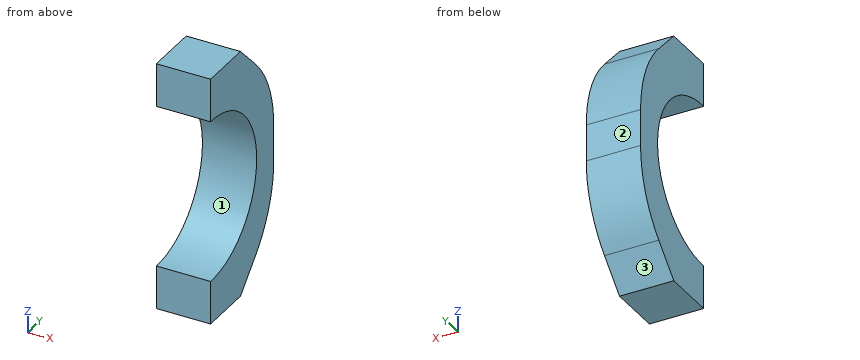
from build123d import *

# Parameters (mm, degrees)
BOSS_EXTRUDE1_DEPTH = 12
CHAMFER1_SIZE       = 16
FILLET1_R           = 30
BOSS_EXTRUDE3_DEPTH = 15


with BuildPart() as part:
    # Sketch1 → Boss-Extrude1 (new body)
    with BuildSketch(Plane(origin=(0, 0, 0), x_dir=(0, 0, -1), z_dir=(1, 0, 0))):
        with BuildLine():
            Line((-33.494680249, 0), (33.494680249, 0))
            Line((33.494680249, 0), (33.494680249, -29.5))
            Line((33.494680249, -29.5), (23.494680249, -29.5))
            ThreePointArc((23.494680249, -29.5), (0, -6.5), (-23.494680249, -29.5))
            Line((-23.494680249, -29.5), (-33.494680249, -29.5))
            Line((-33.494680249, -29.5), (-33.494680249, 0))
        make_face()
    extrude(amount=BOSS_EXTRUDE1_DEPTH)

    # Chamfer1
    chamfer1_edges = [part.edges().sort_by_distance(p)[0] for p in [
        (6, 0, 33.494680249),
        (6, 0, -33.494680249),
    ]]
    chamfer(chamfer1_edges, length=CHAMFER1_SIZE)

    # Fillet1
    fillet1_edges = [part.edges().sort_by_distance(p)[0] for p in [
        (6, 0, 17.494680249),
        (6, 0, -17.494680249),
    ]]
    fillet(fillet1_edges, radius=FILLET1_R)

    # Sketch6 → Boss-Extrude3 (add)
    with BuildSketch(Plane(origin=(12, 0, 0), x_dir=(0, 0, -1), z_dir=(1, 0, 0))):
        with BuildLine():
            Line((34.494680249, -15.585786438), (26.988583595, -8.079689783))
            ThreePointArc((26.988583595, -8.079689783), (16.931459781, -1.359734492), (5.068273378, 1))
            Line((5.068273378, 1), (-5.068273378, 1))
            ThreePointArc((-5.068273378, 1), (-16.931459781, -1.359734492), (-26.988583595, -8.079689783))
            Line((-26.988583595, -8.079689783), (-34.494680249, -15.585786438))
            Line((-34.494680249, -15.585786438), (-34.494680249, -30.5))
            Line((-34.494680249, -30.5), (-22.494443758, -30.5))
            ThreePointArc((-22.494443758, -30.5), (0, -7.5), (22.494443758, -30.5))
            Line((22.494443758, -30.5), (34.494680249, -30.5))
            Line((34.494680249, -30.5), (34.494680249, -15.585786438))
        make_face()
    extrude(amount=-BOSS_EXTRUDE3_DEPTH)


solid = part.part
Check sheet for the modelled part. Datum: model origin and axes. Units: mm. Face numbers are marked on the shaded views. Give positions to 0.01 mm unless a question says otherwise; leave off trailing zeros. Loops run counter-clockwise (first coordinate to the right, second up) from the corner with the lowest first, then second, coordinate; pieces in that order, holes last. Notation, with made-up numbers: M 87,48.5 L 139,48.5 A13 ccw 139,58.5 Z; hole C 28.25,17.25 d10. An arc over 180 degrees is marked long. Answer as a JSON object with one key per item and string values. Group by question number.
Q1. Material ranges on line 1 along Z through (x, y) = (9.75, -12.5); line 2 along Z through (x, y) = (1, -28); line 3 along Y through (x, z) = (2.75, 0), recorded low to high. Write a range as [from, to].
Q2. Cross-section at D-D on z = 0. Record the cut outline in (x, y), then the cut area to 4 significant figures.
Q3. Release check for a two-part mould opening along Z. For the marked faces 1, 2 and 3 record: released by +Z, released by -Z, zero draft, split by the parting line, or undercut.
Q4. Cross-section at C-C on y = -18.5. Record the cut outline in (x, z).
Q5. Cross-section at A-A on y = -10.5. Record the cut outline in (x, z).
Q6. Go/stop test with flat-tipped pins: P1, Ø4, axis at x = -0.5, y = -13, coming from the -Z side; P2, Ø2, axis at x = 3.5, z = 17, coming from the -Y side; P3, Ø2, axis at x = 5, z = 9.5, coming from the -Y side. Record where each tip stops, or that it passes through.
Evaluation:
{
 "1": {"line 1": "z = [-31.41, -14.14], [14.14, 31.41]", "line 2": "z = [-34.49, -22.41], [22.41, 34.49]", "line 3": "y = [-7.5, 1]"},
 "2": {"outline": "M -3,-7.5 L 12,-7.5 L 12,1 L -3,1 Z", "area": "127.5 mm2"},
 "3": {"face 1": "undercut", "face 2": "zero draft", "face 3": "released by -Z"},
 "4": {"outline": "M -3,-34.49 L 12,-34.49 L 12,-19.34 L -3,-19.34 Z; M -3,19.34 L 12,19.34 L 12,34.49 L -3,34.49 Z"},
 "5": {"outline": "M -3,-29.41 L 12,-29.41 L 12,-11.22 L -3,-11.22 Z; M -3,11.22 L 12,11.22 L 12,29.41 L -3,29.41 Z"},
 "6": {"P1": "stops at z = -33.91", "P2": "stops at y = -16.5", "P3": "stops at y = -10.1"}
}
